Work out the finished part from the listing and answer in its coordinate system (mm). Round coordinates to 2 decimals unless told otherwise and drop trailing zeros. Loops run counter-clockwise (first coordinate to the right, second up) from the corner with the lowest first, then second, coordinate; pieces in that order, holes last.
from build123d import *

# Parameters (mm, degrees)
F0_W     = 924
F0_H     = 1510
F0_W_2   = 50
F0_H_2   = 240
F1_DEPTH = 50
F2_DEPTH = 100
F3_DEPTH = 100


with BuildPart() as f1:
    # F0 (on Front) → F1 (new body)
    with BuildSketch(Plane.XZ):
        Polygon((0, 0), (-1024, 0), (-1024, -1610), (-974, -1610), (-50, -1610), (0, -1610), align=None)
        with Locations((-512, -805)):
            Rectangle(F0_W, F0_H, mode=Mode.SUBTRACT)
        with Locations((-999, -1730)):
            Rectangle(F0_W_2, F0_H_2)
        with Locations((-25, -1730)):
            Rectangle(F0_W_2, F0_H_2)
    extrude(amount=F1_DEPTH)

    # F0 (on Front) → F2 (join)
    with BuildSketch(Plane.XZ):
        Polygon((-974, -1850), (-1024, -1850), (-1074, -1850), (-1074, -1870), (-924, -1870), (-924, -1850), align=None)
    extrude(amount=F2_DEPTH)

    # F0 (on Front) → F3 (join)
    with BuildSketch(Plane.XZ):
        Polygon((50, -1850), (0, -1850), (-50, -1850), (-100, -1850), (-100, -1870), (50, -1870), align=None)
    extrude(amount=F3_DEPTH)


solid = f1.part
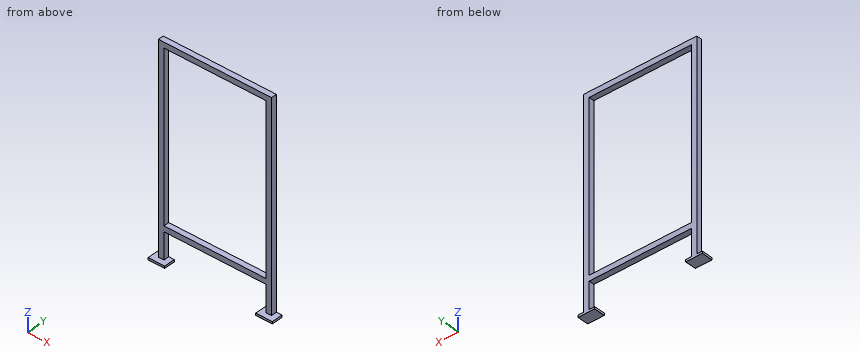
Item 1: Section B-B, the plane z = -491 is taken. Give the vertices of the cut face in (x, y).
Item 2: Straight lines are drawn through the part: line 1 (Z direction, x = -294, y = -4.5); line 2 (X direction, y = -25.5, z = -882); line 3 (Z direction, x = -72, y = -48). For each, find the intervals that lie inside material, in ascending order.
Item 3: Section C-C, the plane x = -956 is taken. Give the vertices of the cut face in (y, z).
Item 4: Section A-A, the plane y = -74 is taken. Give the vertices of the cut face in (x, z), plus the area to 3 significant figures.
Item 5: Each of these flat-tipped pins is pushed along its axis until it touches: P1, Ø8, axis at y = -52, z = -243, coming from the +X side; P2, Ø25, axis at x = -343.5, y = -27, coming from the -Z side; P3, Ø2, axis at y = -36.5, z = -713.5, coming from the -X side. Where does it stop, or does it pass through?
Answer below:
1. outline: (-1024, -50) - (-974, -50) - (-974, 0) - (-1024, 0) - close; (-50, -50) - (0, -50) - (0, 0) - (-50, 0) - close
2. line 1: z = -1610 to -1560, -50 to 0
2. line 2: x = -1024 to -974, -50 to 0
2. line 3: z = -1870 to -1850, -1610 to -1560, -50 to 0
3. outline: (-100, -1870) - (0, -1870) - (0, -1850) - (-100, -1850) - close; (-50, -1610) - (0, -1610) - (0, -1560) - (-50, -1560) - close; (-50, -50) - (0, -50) - (0, 0) - (-50, 0) - close
4. outline: (-1074, -1870) - (-924, -1870) - (-924, -1850) - (-1074, -1850) - close; (-100, -1870) - (50, -1870) - (50, -1850) - (-100, -1850) - close
4. area: 6,000 mm2
5. P1: stops at x = 0
5. P2: stops at z = -1610
5. P3: stops at x = -1024
